Job drawing, mm, ordinate dimensions from the low corner. One solid piece. A direction names the side the tool comes from. Round coordinates to 2 decimals unless told otherwise and drop trailing zeros. Order: outer loops, then holes, each group sorted by start corner. A loop starts at its lowest first (then second) coordinate and runs counter-clockwise, first axis right, second up. Notation, with made-up numbers: (24, 81) -> (32, 81) arc R28 ccw to (32, 101) -> close; hole circle Ø1 at (70.5, 19). An arc over 180 degrees is marked (long way). Write item = value, one per line.
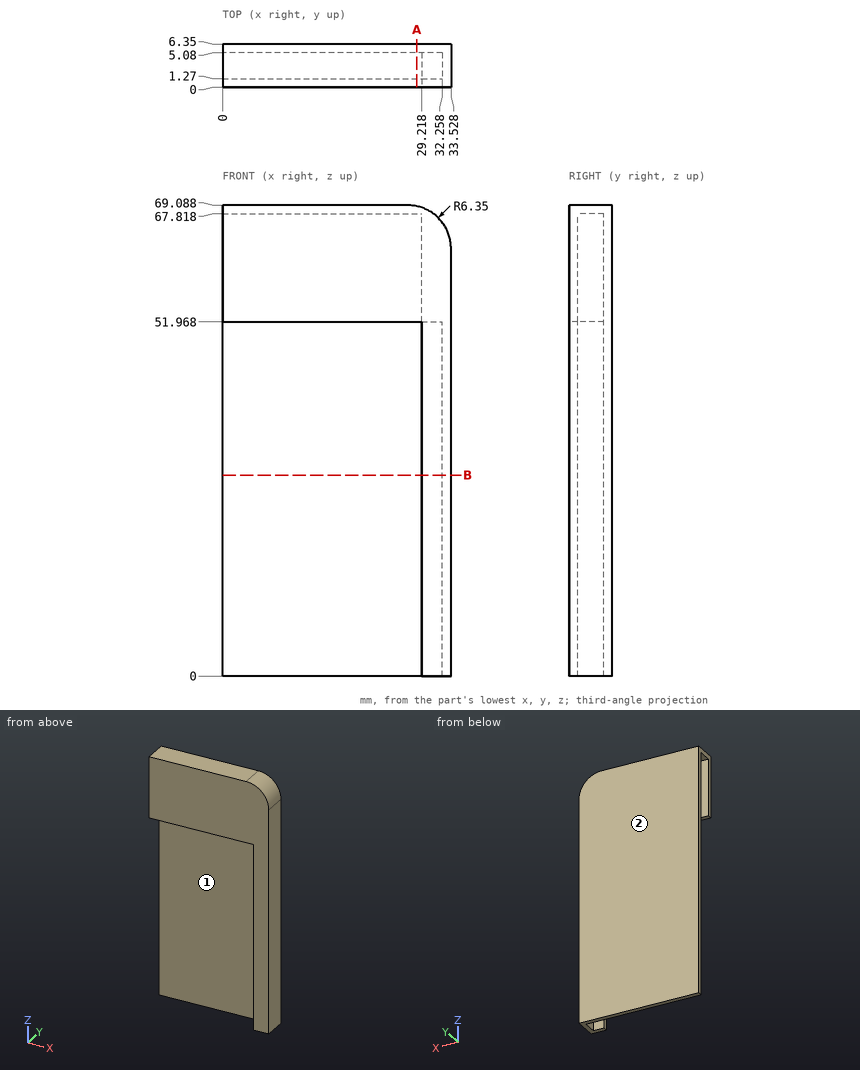
Q1. Probe probe 1 along Y at (x, z) = (24, 57); probe 2 along Y at (x, z) = (26, 31); probe 3 along Z at (x, y) = (27.5, 1.5). List the from-to ranges inside material, lowest first.
Check values:
probe_1 = 0 to 1.27, 5.08 to 6.35
probe_2 = 5.08 to 6.35
probe_3 = 67.82 to 69.08
Q2. Cut at B-B, the plane z = 29.5. List the corners of the cut face in (x, y).
Check values:
outline = (0, 5.08) -> (32.26, 5.08) -> (32.26, 1.27) -> (29.22, 1.27) -> (29.22, 0) -> (33.53, 0) -> (33.53, 6.35) -> (0, 6.35) -> close
Q3. Cut at A-A, the plane x = 28.5. List the corners of the cut face in (y, z).
Check values:
outline = (0, 51.97) -> (1.27, 51.97) -> (1.27, 67.82) -> (5.08, 67.82) -> (5.08, 0) -> (6.35, 0) -> (6.35, 68.95) -> (0, 68.95) -> close
Q4. Which spindle directions (+Z, -Z, +X, -X, +Y, -Y) get a long thin tool onto all of the face, cutting with end or side? Do the marked faces 1 and 2. Say none if no direction does.
Check values:
face_1 = -Z, -X
face_2 = +Z, -Z, +X, -X, +Y
Q5. Flat gauge pins, fed straight in: pin 1 (1.5 mm diameter, centred on y = 5, z = 12, fed in from -X); pin 2 (0.6 mm diameter, centred on x = 18, y = 0.5, fed in from -Z); pin 3 (3 mm diameter, centred on y = 3.5, z = 34, fed in from -X); pin 4 (3 mm diameter, centred on x = 10, y = 3, fed in from -Z). Where does each tip first touch, or does it go through?
Check values:
pin_1 = 0
pin_2 = 51.97
pin_3 = 32.26
pin_4 = 67.82
